Geometry: final body of the model. Coordinates: model frame, mm. Give positions to 0.01 mm unless a question says otherwise; leave off trailing zeros. Loops run counter-clockwise (first coordinate to the right, second up) from the corner with the lowest first, then second, coordinate; pieces in that order, holes last. Notation, with made-up numbers: (60, -21) - (118, -21) arc R23 ccw to (118, 1) - close; hole circle Ø4 at (37.5, 64). An arc over 180 degrees is marked (long way). Answer in a Markdown table with one row per item.
Autodesk Inventor part; units mm, degrees
ref_plane "YZ Plane" through (0, 0, 0) normal (1, 0, 0) x (0, 1, 0)
ref_plane "XZ Plane" through (0, 0, 0) normal (0, 1, 0) x (-1, 0, 0)
ref_plane "XY Plane" through (0, 0, 0) normal (0, 0, 1) x (1, 0, 0)
sketch "Sketch1" plane through (0, 0, 0) normal (0, 1, 0) x (-1, 0, 0)
  circle A0 centre (0, 0) radius 4
  dimension "d0" = 8
extrude "Extrusion1" add sketch "Sketch1" along normal blind 40.5
chamfer "Chamfer1" distance 0.5 angle 45 1 edges at (4, 0, 0)
sketch "Sketch2" plane through (0, 0, 0) normal (0, 0, 1) x (1, 0, 0)
  line L0 (-4, 0.5) -> (-4, 40.5) construction
  line L1 (-3.5, 0) -> (-4, 0.5) construction
  line L2 (-4, 0.5) -> (4, 0.5) construction
  line L3 (3.5, 0) -> (-3.5, 0) construction
  line L4 (4, 40.5) -> (-4, 40.5)
  line L5 (-4, 0.5) -> (4, 0.5) construction
  line L6 (3.5, 0) -> (4, 0.5) construction
  line L7 (4, 0.5) -> (4, 40.5) construction
  line L8 (4, 3) -> (3.5, 3)
  line L9 (3.5, 3) -> (3.5, 2)
  line L10 (3.5, 2) -> (4, 2)
  line L11 (4, 2) -> (4, 3)
  line L12 (0, -7.9) -> (0, 47.4)
  point P0 (0, 0)
  dimension "d6" = 2
  dimension "d7" = 1
  dimension "d8" = 0.5
revolve "Revolution1" cut sketch "Sketch2" angle 360 about axis through (0, -10, 0) along (0, 1, 0)
sketch "Sketch6" plane through (0, 3, 0) normal (0, -1, 0) x (1, 0, 0)
  circle A0 centre (0, 0) radius 3.5 construction
  circle A1 centre (0, 0) radius 4 construction
  circle A2 centre (0, 0) radius 4
  circle A3 centre (0, 4) radius 0.5
extrude "Extrusion4" cut sketch "Sketch6" against normal blind 5 contours A3 A2 | A2 A3 picked at (0.0193, 3.8321) picked at (0.0153, 4.1636)
sketch "Sketch7" plane through (0, 40.5, 0) normal (0, 1, 0) x (1, 0, 0)
  arc A0 (0.499, -3.9688) -> (-0.499, -3.9688) centre (0, -4) ccw
  circle A1 centre (0, -4) radius 0.5
  point P0 (0, 0)
  point P1 (-0.499, -3.9688)
  point P2 (0.499, -3.9688)
extrude "Extrusion5" cut sketch "Sketch7" against normal blind 5
properties part number "Trục"
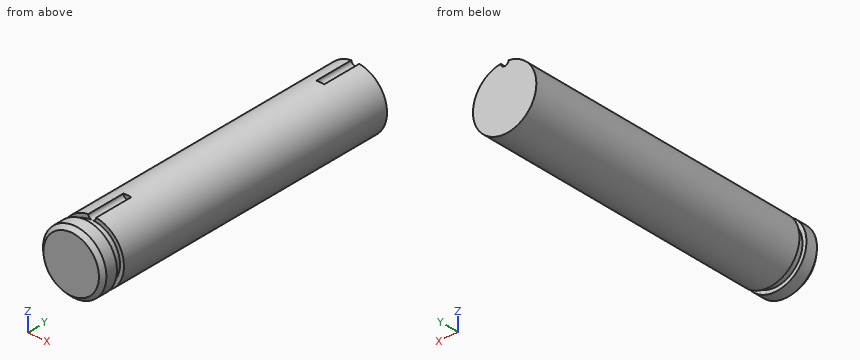
Q1. Cut plane A-A (y = 25). Output: boundary loops of the cut face in (x, z).
Check values:
| item | result |
|---|---|
| outline | circle Ø8 at (0, 0) |
Q2. First-contact query: pin 1 (1.5 mm diameter, centred on x = -3, y = 23, fed in from +Z). Flat tip, straight axial feed; report the tip coordinate or a pass-through.
Check values:
| item | result |
|---|---|
| pin 1 | z = 3.31 |
Q3. Material intervals for line 1 along Z through (x, y) = (-0.25, 20); line 2 along Y through (x, z) = (0.5, 3.5), sorted ascending.
Check values:
| item | result |
|---|---|
| line 1 | -3.99 to 3.99 |
| line 2 | 0.04 to 2, 3 to 40.5 |
